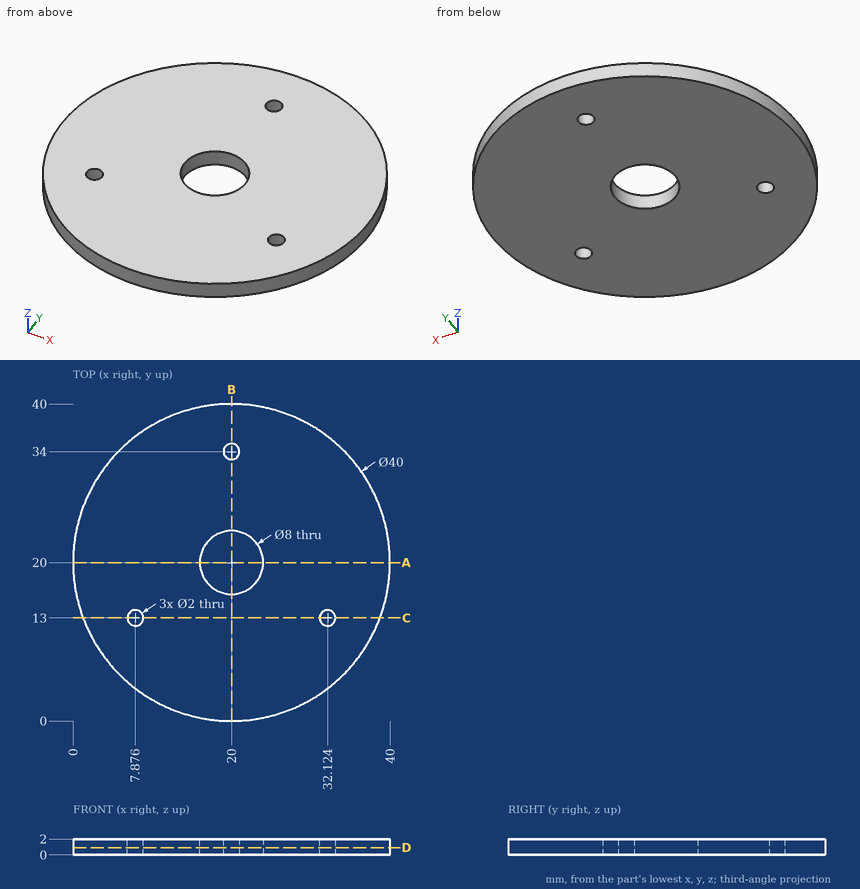
Geometry: see drawing. Coordinates: mm, zero at the bounding-box minimum. Give positions to 0.01 mm unless a question says otherwise; leave off trailing zeros. Order: outer loops, then holes, each group sorted by start corner. A loop starts at its lowest first (then second) coordinate and runs counter-clockwise, first axis right, second up. Notation, with made-up numbers: M 41.5,23.5 L 57.5,23.5 A22 cw 57.5,55.5 Z; hole C 33,12 d8. An arc over 180 degrees is marked long. Answer as CSV lines item,"result". Start each with the question number.
1) Cut plane C-C (y = 13). Output: boundary loops of the cut face in (x, z) (1 decimal).
2) Cut plane B-B (x = 20). Output: boundary loops of the cut face in (y, z).
3) Cut plane A-A (y = 20). Output: boundary loops of the cut face in (x, z).
4) Cut plane D-D (z = 0.9). Output: boundary loops of the cut face in (x, y) (1 decimal), then the cut area to 3 significant figures.
5) Line query: line 1 (Y direction, x = 20, z = 1.2); line 2 (X direction, y = 18, z = 1.55) (1 decimal); line 3 (X direction, y = 18.5, z = 1.85). Output: solid intervals per line, ascending. Write a range as from..to.
6) First-contact query: P1, Ø1, axis at y = 30, z = 1.5, coming from the +X side; P2, Ø1.8, axis at x = 20, y = 34, coming from the -Z side. Flat tips, straight axial feed; report the tip coordinate or a pass-through.
Findings below:
1,outline,"M 1.3,0 L 6.9,0 L 6.9,2 L 1.3,2 Z; M 8.9,0 L 31.1,0 L 31.1,2 L 8.9,2 Z; M 33.1,0 L 38.7,0 L 38.7,2 L 33.1,2 Z"
2,outline,"M 0,0 L 16,0 L 16,2 L 0,2 Z; M 24,0 L 33,0 L 33,2 L 24,2 Z; M 35,0 L 40,0 L 40,2 L 35,2 Z"
3,outline,"M 0,0 L 16,0 L 16,2 L 0,2 Z; M 24,0 L 40,0 L 40,2 L 24,2 Z"
4,outline,"C 20,20 d40; hole C 7.9,13 d2; hole C 20,20 d8; hole C 20,34 d2; hole C 32.1,13 d2"
4,area,"1,200 mm²"
5,line 1,"y = 0..16, 24..33, 35..40"
5,line 2,"x = 0.1..16.5, 23.5..39.9"
5,line 3,"x = 0.06..16.29, 23.71..39.94"
6,P1,"stops at x = 37.6"
6,P2,"passes through"
